```python
from build123d import *

# Parameters (mm, degrees)
SKETCH_1_R      = 7
SKETCH_1_R_2    = 2.5
EXTRUDE_1_DEPTH = 2.5
EXTRUDE_START   = -1
SKETCH_2_R      = 8.5
SKETCH_2_R_2    = 2.5
EXTRUDE_2_DEPTH = 1
CHAMFER_1_SIZE  = 0.2
CHAMFER_2_SIZE  = 0.4


with BuildPart() as part:
    # 草图1 → 凸台-拉伸1 (new, symmetric)
    with BuildSketch(Plane.XY):
        Circle(SKETCH_1_R)
        Circle(SKETCH_1_R_2, mode=Mode.SUBTRACT)
    extrude(amount=EXTRUDE_1_DEPTH, both=True)

    # 草图2 → 凸台-拉伸2 (add)
    with BuildSketch(Plane.XY.offset(2.5).offset(EXTRUDE_START)):
        Circle(SKETCH_2_R)
        Circle(SKETCH_2_R_2, mode=Mode.SUBTRACT)
    extrude(amount=EXTRUDE_2_DEPTH)

    # 倒角1
    chamfer_1_edges = [part.edges().sort_by_distance(p)[0] for p in [
        (-8.5, 0, 2.5),
        (-8.5, 0, 1.5),
        (-7, 0, -2.5),
    ]]
    chamfer(chamfer_1_edges, length=CHAMFER_1_SIZE)

    # 倒角2
    chamfer_2_edges = [part.edges().sort_by_distance(p)[0] for p in [
        (-2.5, 0, -2.5),
        (-2.5, 0, 2.5),
    ]]
    chamfer(chamfer_2_edges, length=CHAMFER_2_SIZE)


solid = part.part
```
Part model, mm, in its own coordinate system. Coordinates: 2 decimals unless noted, no trailing zeros. Order: outer loops, then holes, each group sorted by start corner. A loop starts at its lowest first (then second) coordinate and runs counter-clockwise, first axis right, second up. Notation, with made-up numbers: (46.25, -1) -> (96.25, -1) arc R12 cw to (96.25, 12) -> close; hole circle Ø2 at (38, 62.5). An arc over 180 degrees is marked (long way). Put each result on its own line as item: value. Start each with the question number.
(1) Mould opens along Y. For faces 1 (the face through (-0.54, -2.44, -0.03)), 2 (the face through (6.466, -2.681, -0.373)), 3 (the face through (-4, -6, 1.5)) say: pulls with the +Y half, pulls with the -Y half, needs draft (parallel to the pull), parting line crosses it, or undercut.
(2) Band-saw the part on A-A (x = 0). Give the cut face in (y, z), then the cut area to 3 significant figures.
(3) Probe line 1 along Y through (x, z) = (0, -0.6); line 2 along Z through (x, y) = (4.75, -6.25); line 3 along Y through (x, z) = (2.25, 1.65). List the from-to ranges inside material, lowest first. Write a range as [from, to].
(4) Pin check, flat tips, straight feed: pin 1 Ø1 at (y, z) = (-3, -0.5) entering from +X; pin 2 Ø1.5 at (x, z) = (-1, -1.5) entering from +Y; pin 3 Ø2 at (x, z) = (-4.5, 0) entering from +Y. Stop position of each tip, or through.
(5) Band-saw the part on C-C (z = 0.65). Give the cut face in (x, y), then the cut area to 3 significant figures.
Determined:
1. face 1: undercut
1. face 2: parting line crosses it
1. face 3: needs draft
2. outline: (-8.5, 1.7) -> (-8.3, 1.5) -> (-7, 1.5) -> (-7, -2.3) -> (-6.8, -2.5) -> (-2.9, -2.5) -> (-2.5, -2.1) -> (-2.5, 2.1) -> (-2.9, 2.5) -> (-8.3, 2.5) -> (-8.5, 2.3) -> close; (2.5, -2.1) -> (2.9, -2.5) -> (6.8, -2.5) -> (7, -2.3) -> (7, 1.5) -> (8.3, 1.5) -> (8.5, 1.7) -> (8.5, 2.3) -> (8.3, 2.5) -> (2.9, 2.5) -> (2.5, 2.1) -> close
2. area: 47.6 mm²
3. line 1: y = [-7, -2.5], [2.5, 7]
3. line 2: z = [1.5, 2.5]
3. line 3: y = [-8.14, -1.09], [1.09, 8.14]
4. pin 1: stops at x = 6.54
4. pin 2: stops at y = 7
4. pin 3: stops at y = 6.06
5. outline: circle Ø14 at (0, 0); hole circle Ø5 at (0, 0)
5. area: 134 mm²
